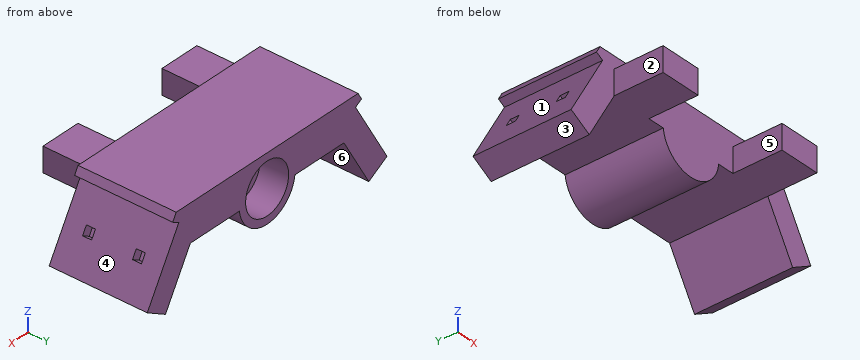
from build123d import *

# Parameters (mm, degrees)
BOSS_EXTRUDE1_DEPTH            = 12
F_2_5_2_5_DIAMETER_HOLE1_D     = 2.5
F_2_5_2_5_DIAMETER_HOLE1_DEPTH = 10
F_2_5_2_5_DIAMETER_HOLE1_TIP   = 0.751075774
SKETCH4_R                      = 3.0762
CUT_EXTRUDE1_DEPTH             = 3.5
SKETCH5_W                      = 5
SKETCH5_H                      = 3
BOSS_EXTRUDE2_DEPTH            = 6
SKETCH7_W                      = 1.1
SKETCH7_H                      = 1.1
CUT_EXTRUDE3_DEPTH             = 1.1
SKETCH8_W                      = 1.1
SKETCH8_H                      = 1.1
CUT_EXTRUDE4_DEPTH             = 1.1


with BuildPart() as part:
    # Sketch1 → Boss-Extrude1 (new body)
    with BuildSketch(Plane(origin=(0, 0, 0), x_dir=(1, 0, 0), z_dir=(0, 1, 0))):
        with BuildLine():
            Line((-13, -4), (13, -4))
            Line((13, -4), (13.5, -3.133974596))
            Line((13.5, -3.133974596), (12.633974596, -2.633974596))
            Line((12.633974596, -2.633974596), (17.133974596, 5.160254038))
            Line((17.133974596, 5.160254038), (14.535898385, 6.660254038))
            Line((14.535898385, 6.660254038), (10.979274058, 0.5))
            Line((10.979274058, 0.5), (3.968626967, 0.5))
            ThreePointArc((3.968626967, 0.5), (0, 4), (-3.968626967, 0.5))
            Line((-3.968626967, 0.5), (-10.979274058, 0.5))
            Line((-10.979274058, 0.5), (-14.535898385, 6.660254038))
            Line((-14.535898385, 6.660254038), (-17.133974596, 5.160254038))
            Line((-17.133974596, 5.160254038), (-12.633974596, -2.633974596))
            Line((-12.633974596, -2.633974596), (-13.5, -3.133974596))
            Line((-13.5, -3.133974596), (-13, -4))
        make_face()
    extrude(amount=BOSS_EXTRUDE1_DEPTH)

    # Ø2.5 (2.5) Diameter Hole1
    with Locations(Plane(origin=(0, 12, 0), x_dir=(1, 0, 0), z_dir=(0, 1, 0))):
        with Locations((0, 0)):
            Hole(F_2_5_2_5_DIAMETER_HOLE1_D / 2, depth=F_2_5_2_5_DIAMETER_HOLE1_DEPTH)
            with Locations((0, 0, -(F_2_5_2_5_DIAMETER_HOLE1_DEPTH + F_2_5_2_5_DIAMETER_HOLE1_TIP / 2))):  # 118° drill point
                Cone(0, F_2_5_2_5_DIAMETER_HOLE1_D / 2, F_2_5_2_5_DIAMETER_HOLE1_TIP, mode=Mode.SUBTRACT)

    # Sketch4 → Cut-Extrude1 (cut)
    with BuildSketch(Plane(origin=(0, 12, 0), x_dir=(1, 0, 0), z_dir=(0, 1, 0))):
        with Locations(Location((0, 0, 0), (0, 0, 270))):
            Circle(SKETCH4_R)
    extrude(amount=-CUT_EXTRUDE1_DEPTH, mode=Mode.SUBTRACT)

    # Sketch5 → Boss-Extrude2 (add)
    with BuildSketch(Plane.XZ):
        with Locations((8.5, 1)):
            Rectangle(SKETCH5_W, SKETCH5_H)
        with Locations((-8.5, 1)):
            Rectangle(SKETCH5_W, SKETCH5_H)
    extrude(amount=BOSS_EXTRUDE2_DEPTH)

    # Sketch7 → Cut-Extrude3 (cut)
    with BuildSketch(Plane(origin=(-10.616025404, 0, 6.129165125), x_dir=(0.49999999999999906, 0, 0.8660254037844393), z_dir=(-0.8660254037844392, 0, 0.499999999999999))):
        with Locations((-8.535898385, 9.05)):
            Rectangle(SKETCH7_W, SKETCH7_H)
        with Locations((-8.535898385, 2.95)):
            Rectangle(SKETCH7_W, SKETCH7_H)
    extrude(amount=-CUT_EXTRUDE3_DEPTH, mode=Mode.SUBTRACT)

    # Sketch8 → Cut-Extrude4 (cut)
    with BuildSketch(Plane(origin=(10.616025404, 0, 6.129165125), x_dir=(0.4999999999999978, 0, -0.86602540378444), z_dir=(0.86602540378444, 0, 0.4999999999999978))):
        with Locations((8.535898385, 9.05)):
            Rectangle(SKETCH8_W, SKETCH8_H)
        with Locations((8.535898385, 2.95)):
            Rectangle(SKETCH8_W, SKETCH8_H)
    extrude(amount=-CUT_EXTRUDE4_DEPTH, mode=Mode.SUBTRACT)


solid = part.part
Can you work these out from the model? Positions are in its coordinate system, mm. Face numbers are marked on the shaded views. A direction names the side the tool comes from. Give positions to 0.01 mm unless a question says otherwise; leave off trailing zeros. Order: outer loops, then holes, each group sorted by start corner. A loop starts at its lowest first (then second) coordinate and runs counter-clockwise, first axis right, second up. Notation, with made-up numbers: M -38.5,2 L -2.5,2 A30 cw -2.5,25 Z; hole C 3,5.25 d11. An arc over 180 degrees is marked long. Use one line per item in the form item = value.
Item 1: For the marked faces 4, 5 and 6, which set-ups out of +Z, -Z, +X, -X, +Y, -Y let a thin tool reach every point of the face, with its end or its side?
Values follow:
face_4 = +X, +Y, -Y
face_5 = +Z, -Z, -Y
face_6 = -Z, +Y, -Y
Item 2: Thinking about a two-plate mould opening in Z: for the marked faces 1, 2 and 3, which applies, pulls with the +Z half, pulls with the -Z half, needs draft (parallel to the pull), parting line crosses it, or undercut?
Values follow:
face_1 = undercut
face_2 = needs draft
face_3 = pulls with the -Z half
Item 3: Will these pins go through, and if not, where does the flat tip stop? pin 1 Ø3.5 at (x, z) = (0, 0) entering from +Y; pin 2 Ø7.5 at (x, y) = (-8, 4.5) entering from -Z; pin 3 Ø1.5 at (y, z) = (-3.5, 1.5) entering from -X.
Values follow:
pin_1 = 8.5
pin_2 = -1.83
pin_3 = -11
Item 4: If we section it at C-C, the plane x = 9: Write out the boundary of the cut face in (y, z), and give its area (3 significant figures).
Values follow:
outline = M -6,-0.5 L 12,-0.5 L 12,4 L 0,4 L 0,2.5 L -6,2.5 Z
area = 72.0 mm^2
Item 5: If we section it at A-A, the plane y = -3.5: Write out the boundary of the cut face in (x, z).
Values follow:
outline = M -11,-0.5 L -6,-0.5 L -6,2.5 L -11,2.5 Z; M 6,-0.5 L 11,-0.5 L 11,2.5 L 6,2.5 Z
Item 6: If we section it at D-D, the plane x = -2: Write out the boundary of the cut face in (y, z).
Values follow:
outline = M 0,-3.46 L 12,-3.46 L 12,-2.34 L 8.5,-2.34 L 8.5,2.34 L 12,2.34 L 12,4 L 0,4 Z
Item 7: If I drill on line 1 along Y through (x, z) = (12.5, 2); line 2 along Y through (x, z) = (-1.5, 0); line 3 along Z through (x, y) = (1, 7.5), over which ranges is the centre line in solid material (lowest first)? Write a range as [from, to].
Values follow:
line_1 = [0, 12]
line_2 = [0, 8.5]
line_3 = [-3.87, -0.75], [0.75, 4]
Item 8: If we section it at B-B, the plane z = -5.5: Write out the boundary of the cut face in (x, y), and give its area (3 significant figures).
Values follow:
outline = M -16.55,0 L -13.87,0 L -13.87,12 L -16.55,12 Z; M 13.87,0 L 16.55,0 L 16.55,12 L 13.87,12 Z
area = 64.3 mm^2
